```python
from build123d import *

# Parameters (mm, degrees)
ESQUISSE1_R        = 1.6
ESQUISSE1_R_2      = 10
BOSS_EXTRU_1_DEPTH = 6
CONG_1_R           = 7.5


with BuildPart() as part:
    # Esquisse1 → Boss.-Extru.1 (new body)
    with BuildSketch(Plane(origin=(0, 0, 0), x_dir=(1, 0, 0), z_dir=(0, 1, 0))):
        with BuildLine():
            Line((-87.5, 25), (-78.620925968, 25))
            ThreePointArc((-78.620925968, 25), (0, 82.5), (78.620925968, 25))
            Line((78.620925968, 25), (87.5, 25))
            Line((87.5, 25), (87.5, -25))
            Line((87.5, -25), (78.620925968, -25))
            ThreePointArc((78.620925968, -25), (0, -82.5), (-78.620925968, -25))
            Line((-78.620925968, -25), (-87.5, -25))
            Line((-87.5, -25), (-87.5, 25))
        make_face()
        with Locations(Location((-53.623111018, 44.995132678, 0), (0, 0, 270))):
            Circle(ESQUISSE1_R, mode=Mode.SUBTRACT)
        with Locations(Location((-44.995132678, 53.623111018, 0), (0, 0, 270))):
            Circle(ESQUISSE1_R, mode=Mode.SUBTRACT)
        with Locations(Location((53.623111018, 44.995132678, 0), (0, 0, 270))):
            Circle(ESQUISSE1_R, mode=Mode.SUBTRACT)
        with Locations(Location((44.995132678, 53.623111018, 0), (0, 0, 270))):
            Circle(ESQUISSE1_R, mode=Mode.SUBTRACT)
        with Locations(Location((44.995132678, -53.623111018, 0), (0, 0, 270))):
            Circle(ESQUISSE1_R, mode=Mode.SUBTRACT)
        with Locations(Location((53.623111018, -44.995132678, 0), (0, 0, 270))):
            Circle(ESQUISSE1_R, mode=Mode.SUBTRACT)
        with Locations(Location((-53.623111018, -44.995132678, 0), (0, 0, 270))):
            Circle(ESQUISSE1_R, mode=Mode.SUBTRACT)
        with Locations(Location((-44.995132678, -53.623111018, 0), (0, 0, 270))):
            Circle(ESQUISSE1_R, mode=Mode.SUBTRACT)
        with Locations(Location((0, 65, 0), (0, 0, 270))):
            Circle(ESQUISSE1_R_2, mode=Mode.SUBTRACT)
        with Locations(Location((0, -65, 0), (0, 0, 90))):
            Circle(ESQUISSE1_R_2, mode=Mode.SUBTRACT)
        with Locations(Location((-73.5, 15, 0), (0, 0, 270))):
            Circle(ESQUISSE1_R, mode=Mode.SUBTRACT)
        with Locations(Location((-73.5, -15, 0), (0, 0, 90))):
            Circle(ESQUISSE1_R, mode=Mode.SUBTRACT)
        with Locations(Location((-43.5, 15, 0), (0, 0, 270))):
            Circle(ESQUISSE1_R, mode=Mode.SUBTRACT)
        with Locations(Location((-43.5, -15, 0), (0, 0, 90))):
            Circle(ESQUISSE1_R, mode=Mode.SUBTRACT)
        with Locations(Location((-13.5, 15, 0), (0, 0, 270))):
            Circle(ESQUISSE1_R, mode=Mode.SUBTRACT)
        with Locations(Location((-13.5, -15, 0), (0, 0, 90))):
            Circle(ESQUISSE1_R, mode=Mode.SUBTRACT)
        with Locations(Location((13.5, -15, 0), (0, 0, 270))):
            Circle(ESQUISSE1_R, mode=Mode.SUBTRACT)
        with Locations(Location((13.5, 15, 0), (0, 0, 90))):
            Circle(ESQUISSE1_R, mode=Mode.SUBTRACT)
        with Locations(Location((43.5, 15, 0), (0, 0, 90))):
            Circle(ESQUISSE1_R, mode=Mode.SUBTRACT)
        with Locations(Location((43.5, -15, 0), (0, 0, 270))):
            Circle(ESQUISSE1_R, mode=Mode.SUBTRACT)
        with Locations(Location((73.5, -15, 0), (0, 0, 270))):
            Circle(ESQUISSE1_R, mode=Mode.SUBTRACT)
        with Locations(Location((73.5, 15, 0), (0, 0, 90))):
            Circle(ESQUISSE1_R, mode=Mode.SUBTRACT)
    extrude(amount=BOSS_EXTRU_1_DEPTH)

    # Congé1
    cong_1_edges = [part.edges().sort_by_distance(p)[0] for p in [
        (-78.620925968, 3, -25),
        (78.620925968, 3, -25),
        (78.620925968, 3, 25),
        (-78.620925968, 3, 25),
    ]]
    fillet(cong_1_edges, radius=CONG_1_R)


solid = part.part
```
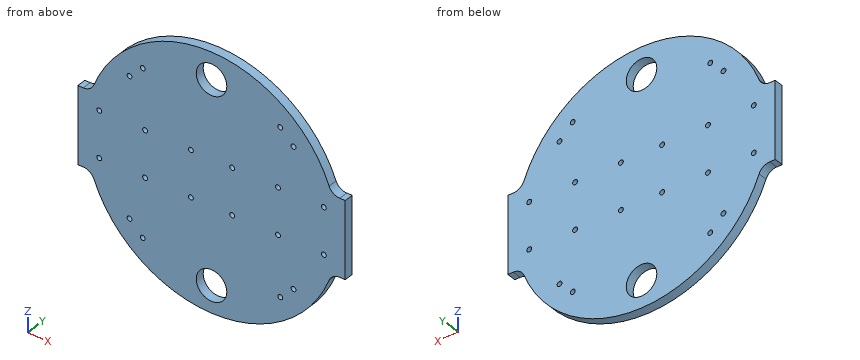
Geometry: final body of the model. Coordinates: model frame, mm. Coordinates: 2 decimals unless noted, no trailing zeros. Order: outer loops, then holes, each group sorted by start corner. A loop starts at its lowest first (then second) coordinate and runs counter-clockwise, first axis right, second up. Notation, with made-up numbers: (6.25, 16) - (47.25, 16) arc R34 cw to (47.25, 52) - close; hole circle Ø2 at (-32.75, 49). An arc over 180 degrees is marked (long way). Write each question's results on one line, items separated by ' | '.
1) Section A-A, the plane z = -65. Return loops of the section in (x, y), plus the area to 3 significant figures.
Results list:
outline: (-50.81, 0) - (-10, 0) - (-10, 6) - (-50.81, 6) - close; (10, 0) - (50.81, 0) - (50.81, 6) - (10, 6) - close | area: 490 mm^2
2) Line query: line 1 (Z direction, x = 73.5, y = 4.85); line 2 (X direction, y = 2.3, z = 65); line 3 (Z direction, x = 66.5, y = 5.5). Output: solid intervals per line, ascending. Write a range as from..to.
Results list:
line 1: -37.47..-16.6, -13.4..13.4, 16.6..37.47 | line 2: -50.81..-10, 10..50.81 | line 3: -48.83..48.83
3) Section D-D, the plane x = -60. Return loops of the section in (y, z).
Results list:
outline: (0, -56.62) - (6, -56.62) - (6, 56.62) - (0, 56.62) - close
4) Pin query (flat end, axial travel): pin 1 (3.5 mm diameter, centred on x = 13.5, z = -15, fed in from -Y); pin 2 (1.8 mm diameter, centred on x = 85.5, y = 2.5, fed in from -Z); pin 3 (3 mm diameter, centred on y = 3.5, z = -52.5, fed in from -X). Return the tip coordinate at first contact, or that it passes through.
Results list:
pin 1: y = 0 | pin 2: z = -25 | pin 3: x = -64.85
5) Section B-B, the plane y = 4.7. State how many separate pieces and enclosed holes the cut face has, plus the area to 3 significant figures.
Results list:
separate pieces: 1 | enclosed holes: 22 | area: 21,200 mm^2
6) Section C-C, the plane z = 70.5. Return loops of the section in (x, y), plus the area to 3 significant figures.
Results list:
outline: (-42.85, 0) - (-8.35, 0) - (-8.35, 6) - (-42.85, 6) - close; (8.35, 0) - (42.85, 0) - (42.85, 6) - (8.35, 6) - close | area: 414 mm^2
